from build123d import *

# Parameters (mm, degrees)
F0_W      = 116
F0_H      = 17
F1_DEPTH  = 2
F2_W      = 17
F2_H      = 2
F3_DEPTH  = 2.2
F5_W      = 3
F5_H      = 6
F6_DEPTH  = 25
F8_DEPTH  = 14
F9_R      = 0.8
F10_R     = 2
F10_R_2   = 3.6
F11_DEPTH = 2


with BuildPart() as f1:
    # F0 (on Top) → F1 (new body)
    with BuildSketch(Plane.XY):
        with Locations((0, 8.5)):
            Rectangle(F0_W, F0_H)
    extrude(amount=F1_DEPTH)

    # F4: F3 across plane


with BuildPart() as f3:
    # F2 (on face) → F3 (new body)
    with BuildSketch(Plane(origin=(-58, 0, 0), x_dir=(0, -1, 0), z_dir=(-1, 0, 0))):
        Polygon((-17, 0), (-17, 2), (-26, 2), (-26, -12), (-17, -12), align=None)
        with Locations((-8.5, 1)):
            Rectangle(F2_W, F2_H)
        Polygon((0, 0), (-17, 0), (-17, -12), (-17, -24), (0, -24), align=None)
    extrude(amount=F3_DEPTH)


with BuildPart() as f1_1:
    add(f1.part)
    add(f3.part.mirror(Plane.YZ))

    # F5 (on face) → F6 (cut)
    with BuildSketch(Plane.XY.offset(2)):
        with Locations((-56.5, 14)):
            Rectangle(F5_W, F5_H)
        with Locations((56.5, 14)):
            Rectangle(F5_W, F5_H)
    extrude(amount=-F6_DEPTH, mode=Mode.SUBTRACT)


    add(f3.part)  # F8 merges F3
    # F7 (on face) → F8 (join, through all)
    with BuildSketch(Plane.XY.offset(2)):
        Polygon((-55, 19.6), (-58, 22.6), (-58, 19.6), align=None)
        Polygon((58, 19.6), (58, 22.6), (55, 19.6), align=None)
    extrude(amount=-F8_DEPTH)

    # F9
    f9_edges = [f1_1.edges().sort_by_distance(p)[0] for p in [
        (55, 19.6, -5),
        (-55, 19.6, -5),
        (58, 19.6, -5),
        (-58, 19.6, -5),
        (-58, 22.6, -5),
        (58, 22.6, -5),
    ]]
    fillet(f9_edges, radius=F9_R)

    # F10 (on face) → F11 (join)
    with BuildSketch(Plane.XZ):
        Polygon((-58, 0), (-58, -24), (-45.2, -24), (-45.2, -9), (-35.2, -9), (-35.2, -24), (58, -24), (58, 0), align=None)
        with Locations((-29, -20)):
            Circle(F10_R, mode=Mode.SUBTRACT)
        with Locations((-19.5, -20)):
            Circle(F10_R, mode=Mode.SUBTRACT)
        with Locations((-10, -20)):
            Circle(F10_R, mode=Mode.SUBTRACT)
        with Locations((-0.5, -20)):
            Circle(F10_R, mode=Mode.SUBTRACT)
        with Locations((9, -20)):
            Circle(F10_R, mode=Mode.SUBTRACT)
        with Locations((18.5, -20)):
            Circle(F10_R, mode=Mode.SUBTRACT)
        with Locations((28, -20)):
            Circle(F10_R, mode=Mode.SUBTRACT)
        with Locations((37.5, -20)):
            Circle(F10_R, mode=Mode.SUBTRACT)
        with Locations((47, -20)):
            Circle(F10_R, mode=Mode.SUBTRACT)
        with Locations((-29, -10)):
            Circle(F10_R_2, mode=Mode.SUBTRACT)
        with Locations((-19.5, -10)):
            Circle(F10_R_2, mode=Mode.SUBTRACT)
        with Locations((-10, -10)):
            Circle(F10_R_2, mode=Mode.SUBTRACT)
        with Locations((-0.5, -10)):
            Circle(F10_R_2, mode=Mode.SUBTRACT)
        with Locations((9, -10)):
            Circle(F10_R_2, mode=Mode.SUBTRACT)
        with Locations((18.5, -10)):
            Circle(F10_R_2, mode=Mode.SUBTRACT)
        with Locations((28, -10)):
            Circle(F10_R_2, mode=Mode.SUBTRACT)
        with Locations((37.5, -10)):
            Circle(F10_R_2, mode=Mode.SUBTRACT)
        with Locations((47, -10)):
            Circle(F10_R_2, mode=Mode.SUBTRACT)
        Polygon((60.2, 2), (-60.2, 2), (-60.2, -24), (-58, -24), (-58, 0), (58, 0), (58, -24), (60.2, -24), align=None)
    extrude(amount=F11_DEPTH)


solid = f1_1.part
Could you check a few things on this model? Use its own coordinates, in mm. A direction names the side the tool comes from. Coordinates: 2 decimals unless noted, no trailing zeros. Write each loop counter-clockwise with the first axis right and the second up, starting at its lowest first coordinate (ties: lowest second). Pieces come first, ordered by that corner, then holes. Notation, with made-up numbers: (4.25, 77) - (19.25, 77) arc R18 ccw to (19.25, 107) - close; hole circle Ø4 at (30, 26.25). An arc over 180 degrees is marked (long way). Put each result on its own line as item: value. Start each with the question number.
Q1. I want a section at A-A on x = -10. Write out the boundary of the cut face in (y, z).
Q2. I'm going to push flat-ended pins straight in: P1, Ø1.5, axis at x = 26, y = 19.5, coming from the +Z side; P2, Ø8.5, axis at x = 25.5, y = 10.5, coming from the -Z side; P3, Ø8.5, axis at x = 18.5, z = -10, coming from the -Y side; P4, Ø8.5, axis at x = 9, z = -10, coming from the +Y side. Where does each tip first touch, or does it pass through?
Q3. Thinking about a two-plate mould opening in X: for faces 4 (the flat face through (58, 10, -11)), 5 (the flat face through (-58.3, 4.7, -24)), which applies, pulls with the +X half, pulls with the -X half, needs draft (parallel to the pull), parting line crosses it, or undercut?
Q4. I want a section at B-B on z = -14.75. Write out the boundary of the cut face in (x, y), plus the area to 3 significant figures.
Q5. Which directions (+Z, -Z, +X, -X, +Y, -Y) give clear straight access to the entire face, cutting with the end or side of a thin tool? Please do faces 1 (the flat face through (-1, 17, 1)), 2 (the flat face through (56, 11, 1)), 3 (the flat face through (-35.2, -1, -16)).
Q6. I want a section at C-C on y = 8.5. Write out the boundary of the cut face in (x, z), plus the area to 3 significant figures.
Q7. Please list where these lines run through material, in increasing order: L1, parallel to Z at x = 28, y = -1.55; L2, parallel to X at y = 2.5, z = -0.25; L3, parallel to Y at x = -26.5, z = -13.75.
Q8. I want a section at D-D on z = -20. Count the separate pieces of the cut face and the enclosed holes in it, plus the area to 3 significant figures.
Checks:
1. outline: (-2, -24) - (0, -24) - (0, -22) - (-2, -22) - close; (-2, -18) - (0, -18) - (0, -13.6) - (-2, -13.6) - close; (-2, -6.4) - (0, -6.4) - (0, 0) - (17, 0) - (17, 2) - (-2, 2) - close
2. P1: through
2. P2: z = 0
2. P3: y = -2
2. P4: y = 0
3. face 4: undercut
3. face 5: needs draft
4. outline: (-60.2, -2) - (-45.2, -2) - (-45.2, 0) - (-58, 0) - (-58, 17) - (-60.2, 17) - close; (-35.2, -2) - (60.2, -2) - (60.2, 17) - (58, 17) - (58, 0) - (-35.2, 0) - close
4. area: 296 mm²
5. face 1: +Z, -Z, +Y
5. face 2: +Z, -Z
5. face 3: -Z, +Y, -Y
6. outline: (-60.2, -24) - (-58, -24) - (-58, 0) - (58, 0) - (58, -24) - (60.2, -24) - (60.2, 2) - (-60.2, 2) - close
6. area: 346 mm²
7. L1: -24 to -22, -18 to -13.6, -6.4 to 2
7. L2: -60.2 to -58, 58 to 60.2
7. L3: -2 to 0
8. separate pieces: 11
8. enclosed holes: 0
8. area: 224 mm²
